Part model, mm, in its own coordinate system. Face numbers are marked on the shaded views. A direction names the side the tool comes from. Coordinates: 2 decimals unless noted, no trailing zeros. Order: outer loops, then holes, each group sorted by start corner. A loop starts at its lowest first (then second) coordinate and runs counter-clockwise, first axis right, second up. Notation, with made-up numbers: (33.5, 71.5) - (89.5, 71.5) arc R28 ccw to (89.5, 98.5) - close; hole circle Ø6 at (83.25, 69.5). An arc over 180 degrees is marked (long way). Use a Markdown table: item, result. Add a question column.
1) Saw through at A-A on x = 17. List the corners of the cut face in (y, z), then the cut area to 3 significant figures.
2) Tool access for the marked faces 1 and 2: list every direction of +Z, -Z, +X, -X, +Y, -Y with a clear straight run to the whole face (end or side of a thin tool).
3) Drop flat-ended pins along their axis: P1, Ø1, axis at x = 35.5, z = 2, coming from the -Y side; P2, Ø4, axis at x = 42.5, z = 5.5, coming from the +Y side; P3, Ø5, axis at x = 21, z = -4.5, coming from the -Y side. Give the stop position or say it passes through.
4) Wall check: L1, parallel to X at y = -6, z = 1.25; L2, parallel to Y at x = 38, z = 0.25; L3, parallel to Z at x = 43, y = 6. Give the ranges that are in metal, low to high. Write a range as [from, to].
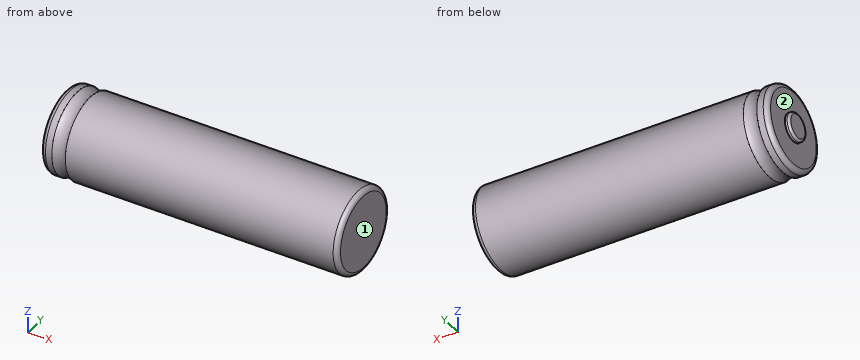
```python
from build123d import *

# Parameters (mm, degrees)
F0_R     = 9
F1_DEPTH = 65.2
F2_R     = 1
F3_R     = 3
F4_DEPTH = 1
F5_R     = 0.5
F6_R     = 3


with BuildPart() as f1:
    # F0 (on Right) → F1 (new body)
    with BuildSketch(Plane.YZ):
        Circle(F0_R)
    extrude(amount=F1_DEPTH)

    # F2
    f2_edges = [f1.edges().sort_by_distance(p)[0] for p in [
        (65.2, -9, 0),
        (0, -9, 0),
    ]]
    fillet(f2_edges, radius=F2_R)

    # F3 (on Right) → F4 (join)
    with BuildSketch(Plane.YZ):
        Circle(F3_R)
    extrude(amount=-F4_DEPTH)

    # F5
    f5_edges = [f1.edges().sort_by_distance(p)[0] for p in [
        (-1, -3, 0),
    ]]
    fillet(f5_edges, radius=F5_R)

    # F6 (on Front) → F7 (revolve, cut)
    with BuildSketch(Plane.XZ):
        with Locations((3.8806945086, 11.6108693182)):
            Circle(F6_R)
    revolve(axis=Axis((1, 0, 0), (1, 0, 0)), mode=Mode.SUBTRACT)


solid = f1.part
```
Results are:
| question | item | result |
|---|---|---|
| 1 | outline | circle Ø18 at (0, 0) |
| 1 | area | 254 mm2 |
| 2 | face 1 | +Z, -Z, +X, +Y, -Y |
| 2 | face 2 | -X |
| 3 | P1 | y = -8.87 |
| 3 | P2 | y = 8.29 |
| 3 | P3 | y = -8.77 |
| 4 | L1 | [0, 65.2] |
| 4 | L2 | [-9, 9] |
| 4 | L3 | [-6.71, 6.71] |
